```python
from build123d import *

# Parameters (mm, degrees)
SKICA8_R                 = 4.5
SKICA8_R_2               = 1.5
P_IDAT_VYSUNUT_M8_DEPTH  = 20
SKICA9_W                 = 8.6
SKICA9_H                 = 1.884529933
ZKOSEN_1_SIZE            = 0.6
ZKOSEN_1_SIZE2           = 1.039230485
ZKOSEN_2_SIZE            = 0.6
ZKOSEN_2_SIZE2           = 1.039230485
ZKOSEN_3_SIZE            = 0.3
SKICA10_R                = 1.5
ODEBRAT_VYSUNUT_M1_DEPTH = 10
SKICA11_R                = 2
ODEBRAT_VYSUNUT_M2_DEPTH = 10


with BuildPart() as part:
    # Skica8 → Přidat vysunutím8 (new body)
    with BuildSketch(Plane(origin=(23.8, 0, 0), x_dir=(1, 0, 0), z_dir=(0, 0, 1))):
        with Locations((-23.8, 0)):
            Circle(SKICA8_R)
        with Locations((-23.8, 0)):
            Circle(SKICA8_R_2, mode=Mode.SUBTRACT)
    extrude(amount=P_IDAT_VYSUNUT_M8_DEPTH)

    # Skica9 → Odebrat rotací1 (revolve, cut)
    with BuildSketch(Plane(origin=(0, 0, 0), x_dir=(0, 0, -1), z_dir=(1, 0, 0))):
        with Locations((-10, 4.392264967)):
            Rectangle(SKICA9_W, SKICA9_H)
    revolve(axis=Axis((0, 0, 0), (0, 0, 1)), mode=Mode.SUBTRACT)

    # Zkosení1
    zkosen_1_edges = [part.edges().sort_by_distance(p)[0] for p in [
        (0, -3.45, 5.7),
    ]]
    zkosen_1_side = [part.faces().sort_by_distance(p)[0] for p in [
        (0, -3.45, 10),
    ]]
    chamfer(zkosen_1_edges, length=ZKOSEN_1_SIZE, length2=ZKOSEN_1_SIZE2, reference=zkosen_1_side[0])

    # Zkosení2
    zkosen_2_edges = [part.edges().sort_by_distance(p)[0] for p in [
        (0, -3.45, 14.3),
    ]]
    zkosen_2_side = [part.faces().sort_by_distance(p)[0] for p in [
        (0, -3.45, 10.3),
    ]]
    chamfer(zkosen_2_edges, length=ZKOSEN_2_SIZE, length2=ZKOSEN_2_SIZE2, reference=zkosen_2_side[0])

    # Zkosení3
    zkosen_3_edges = [part.edges().sort_by_distance(p)[0] for p in [
        (-4.5, 0, 0),
        (-4.5, 0, 20),
    ]]
    chamfer(zkosen_3_edges, length=ZKOSEN_3_SIZE)

    # Skica10 → Odebrat vysunutím1 (cut, symmetric)
    with BuildSketch(Plane(origin=(0, 0, 0), x_dir=(1, 0, 0), z_dir=(0, 1, 0))):
        with Locations((0, -3)):
            Circle(SKICA10_R)
        with Locations((0, -17)):
            Circle(SKICA10_R)
    extrude(amount=ODEBRAT_VYSUNUT_M1_DEPTH, both=True, mode=Mode.SUBTRACT)

    # Skica11 → Odebrat vysunutím2 (cut)
    with BuildSketch(Plane.XY.offset(20)):
        Circle(SKICA11_R)
    extrude(amount=-ODEBRAT_VYSUNUT_M2_DEPTH, mode=Mode.SUBTRACT)


solid = part.part
```
The listing builds one solid part. Answer for the finished solid, in the listing's coordinates (mm). A direction names the side the tool comes from. Round coordinates to 2 decimals unless told otherwise and drop trailing zeros. Loops run counter-clockwise (first coordinate to the right, second up) from the corner with the lowest first, then second, coordinate; pieces in that order, holes last. Notation, with made-up numbers: (0, -36.5) - (17, -36.5) arc R29 cw to (17, -7.5) - close; hole circle Ø9 at (56.5, -21). An arc over 180 degrees is marked (long way). Use one line per item in the form item = value. Start each with the question number.
1. The part is cut by section A-A on z = 17. Determine the outline of the cut face in (x, y), then the cut area to 3 significant figures.
2. The part is cut by section B-B on x = -1.25. Give the number of separate pieces and of enclosed holes in the cut face, then the cut area to 3 significant figures.
3. Given pin 1 Ø3.5 at (x, z) = (0, 17) entering from +Y; pin 2 Ø1.2 at (x, y) = (0.5, -1) entering from +Z; pin 3 Ø4 at (x, z) = (-2.5, 10.5) entering from +Y; pin 4 Ø1.5 at (y, z) = (-2.5, 8.5) entering from +X, each flat-ended and moving along its own axis, determine where each tip first touches the part or whether it passes through.
4. For a pull along Z with two mould halves and no side action, classify faces 3 (the face through (1.321, 3.187, 9.948)), 4 (the face through (2, -1, 20)), 5 (the face through (2, 0, 0)), 6 (the face through (0.806, 2.935, 15.735)) as pulls with the +Z half, pulls with the -Z half, needs draft (parallel to the pull), parting line crosses it, or undercut.
5. A tool of negligible diameter and unlimited length cuts with its end or side. For faces 1 (the face through (-2, 0, 15)), 2 (the face through (-1.5, -2.72, 2.93)), from which of +Z, -Z, +X, -X, +Y, -Y can it reach the whole face along a straight path? Write none if from no direction.
6. Consider line 1 (Z direction, x = 0, y = 3.4); line 2 (Y direction, x = 0, z = 1.05). Determine where each line is inside the solid, lowest interval first. Write a range as [from, to].
7. The part is cut by section C-C on z = 10.5. Determine the outline of the cut face in (x, y).
Geometry check:
q1.outline = (-1.5, -4.24) - (-1.5, -1.32) arc R2 cw to (-1.5, 1.32) - (-1.5, 4.24) arc R4.5 ccw to start; (1.5, -4.24) arc R4.5 ccw to (1.5, 4.24) - (1.5, 1.32) arc R2 cw to (1.5, -1.32) - close
q1.area = 35.3 mm^2
q2.separate_pieces = 6
q2.enclosed_holes = 0
q2.area = 86.4 mm^2
q3.pin_1 = 4.5
q3.pin_2 = 10
q3.pin_3 = 3.41
q3.pin_4 = 2.97
q4.face_3 = undercut
q4.face_4 = pulls with the +Z half
q4.face_5 = pulls with the -Z half
q4.face_6 = undercut
q5.face_1 = +Z
q5.face_2 = +Y, -Y
q6.line_1 = [0, 1.5], [4.5, 15.5], [18.5, 20]
q6.line_2 = [-4.5, -1.5], [1.5, 4.5]
q7.outline = circle Ø6.9 at (0, 0); hole circle Ø4 at (0, 0)
